Part print with two shaded views. Sizes in mm from the minimum x, y, z corner. Round coordinates to 2 decimals unless told otherwise and drop trailing zeros. Loops run counter-clockwise (first coordinate to the right, second up) from the corner with the lowest first, then second, coordinate; pieces in that order, holes last. Notation, with made-up numbers: (52, 45) - (100, 45) arc R7 cw to (100, 52) - close; hole circle Ø5 at (68.25, 83). An arc over 180 degrees is marked (long way). Use a Markdown table: item, result.
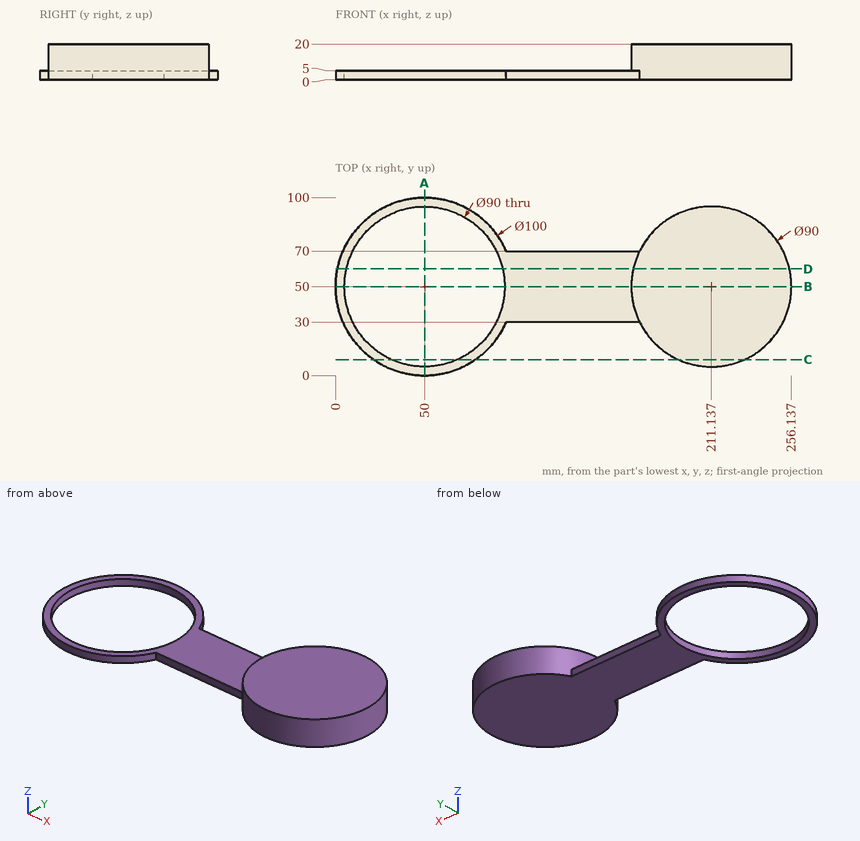
Q1. Drop flat-ended pins along their axis: pin 1 (1.5 mm diameter, centred on x = 145, z = 2, fed in from -Y); pin 2 (6 mm diameter, centred on y = 52.5, z = 16.5, fed in from -X); pin 3 (6 mm diameter, centred on x = 163.5, z = 3.5, fed in from +Y); pin 4 (3 mm diameter, centred on x = 93, z = 8, fed in from +Y). Give the stop position or say it passes through.
Results found:
| item | result |
|---|---|
| pin 1 | stops at y = 30 |
| pin 2 | stops at x = 166.14 |
| pin 3 | stops at y = 70 |
| pin 4 | passes through |
Q2. Cut at D-D, the plane y = 60. List the corners of the cut face in (x, z).
Results found:
| item | result |
|---|---|
| outline | (1.01, 0) - (6.13, 0) - (6.13, 5) - (1.01, 5) - close; (93.87, 0) - (255.01, 0) - (255.01, 20) - (167.26, 20) - (167.26, 5) - (93.87, 5) - close |
Q3. Cut at B-B, the plane y = 50. List the corners of the cut face in (x, z), plus the area to 3 significant figures.
Results found:
| item | result |
|---|---|
| outline | (0, 0) - (5, 0) - (5, 5) - (0, 5) - close; (95, 0) - (256.14, 0) - (256.14, 20) - (166.14, 20) - (166.14, 5) - (95, 5) - close |
| area | 2,180 mm2 |
Q4. Cut at C-C, the plane y = 9. List the corners of the cut face in (x, z).
Results found:
| item | result |
|---|---|
| outline | (21.38, 0) - (31.45, 0) - (31.45, 5) - (21.38, 5) - close; (68.55, 0) - (78.62, 0) - (78.62, 5) - (68.55, 5) - close; (192.59, 0) - (229.68, 0) - (229.68, 20) - (192.59, 20) - close |
Q5. Cut at A-A, the plane x = 50. List the corners of the cut face in (y, z).
Results found:
| item | result |
|---|---|
| outline | (0, 0) - (5, 0) - (5, 5) - (0, 5) - close; (95, 0) - (100, 0) - (100, 5) - (95, 5) - close |
Q6. Probe line 1 (Y direction, x = 50, z = 2.6); line 2 (X direction, y = 12, z = 1.5); line 3 (X direction, y = 79.5, z = 2.25). List the from-to ranges inside material, lowest first.
Results found:
| item | result |
|---|---|
| line 1 | y = 0 to 5, 95 to 100 |
| line 2 | x = 17.5 to 25.9, 74.1 to 82.5, 187.03 to 235.24 |
| line 3 | x = 9.63 to 16.02, 83.98 to 90.37, 177.16 to 245.12 |
